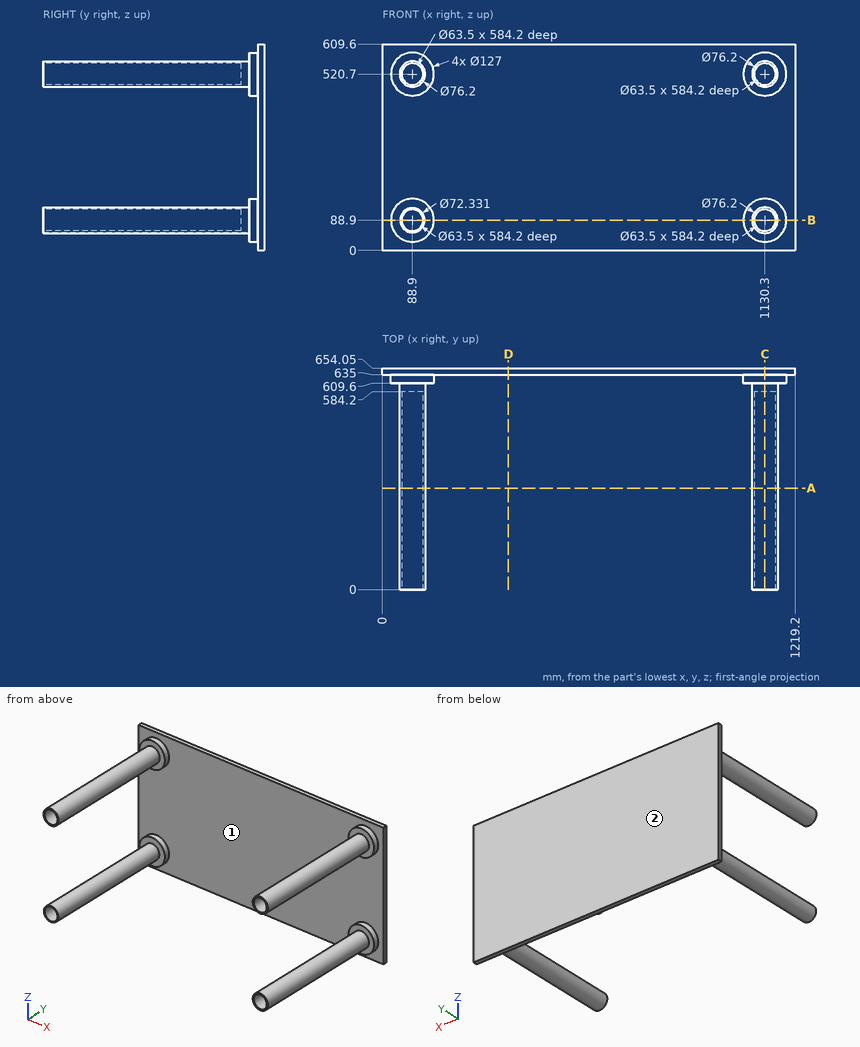
The figure shows three views and two pictorial views of one solid part (mm, origin at its lowest corner). Answer the questions. Coordinates: 2 decimals unless noted, no trailing zeros. Write each loop counter-clockwise with the first axis right and the second up, starting at its lowest first coordinate (ties: lowest second). Pieces come first, ordered by that corner, then holes. Notation, with made-up numbers: (74.5, 47) -> (82.5, 47) arc R14 cw to (82.5, 54) -> close; hole circle Ø10 at (52.25, 24). An arc over 180 degrees is marked (long way). Return JSON: item names as keys, results as strings.
(1) Consider line 1 along X through (y, z) = (209, 520); line 2 along Z through (x, y) = (88, 160); line 3 along Z through (x, y) = (1130.3, 406). Determine where each line is inside the solid, lowest interval first. Write a range as from..to.
Answers below:
{"line 1": "50.81..57.16, 120.64..126.99, 1092.21..1098.56, 1162.04..1168.39", "line 2": "52.75..57.16, 120.64..125.05, 482.61..488.96, 552.44..558.79", "line 3": "50.8..57.15, 120.65..127, 482.6..488.95, 552.45..558.8"}
(2) For a pull along X with two mould halves and no side action, classify the marked faces 1 and 2 as pulls with the +X half, pulls with the -X half, needs draft (parallel to the pull), parting line crosses it, or undercut.
Answers below:
{"face 1": "undercut", "face 2": "needs draft"}
(3) The part is cut by section C-C on x = 1130.3. Give the vertices of the cut face in (y, z), then the cut area to 3 significant figures.
Answers below:
{"outline": "(0, 50.8) -> (609.6, 50.8) -> (609.6, 25.4) -> (635, 25.4) -> (635, 0) -> (654.05, 0) -> (654.05, 609.6) -> (635, 609.6) -> (635, 584.2) -> (609.6, 584.2) -> (609.6, 558.8) -> (0, 558.8) -> (0, 552.45) -> (584.2, 552.45) -> (584.2, 488.95) -> (0, 488.95) -> (0, 482.6) -> (609.6, 482.6) -> (609.6, 457.2) -> (635, 457.2) -> (635, 152.4) -> (609.6, 152.4) -> (609.6, 127) -> (0, 127) -> (0, 120.65) -> (584.2, 120.65) -> (584.2, 57.15) -> (0, 57.15) -> close", "area": "36,800 mm^2"}
(4) The part is cut by section A-A on y = 300. Give the vertices of the cut face in (x, z), then the cut area to 3 significant figures.
Answers below:
{"outline": "circle Ø76.2 at (88.9, 520.7); circle Ø72.33 at (88.9, 88.9); circle Ø76.2 at (1130.3, 88.9); circle Ø76.2 at (1130.3, 520.7); hole circle Ø63.5 at (88.9, 88.9); hole circle Ø63.5 at (88.9, 520.7); hole circle Ø63.5 at (1130.3, 88.9); hole circle Ø63.5 at (1130.3, 520.7)", "area": "5,120 mm^2"}
(5) The part is cut by section D-D on x = 372. Give the vertices of the cut face in (y, z), then the cut area to 3 significant figures.
Answers below:
{"outline": "(635, 0) -> (654.05, 0) -> (654.05, 609.6) -> (635, 609.6) -> close", "area": "11,600 mm^2"}
(6) Each of these flat-tipped pins is pushed along its axis until it touches: P1, Ø19, axis at x = 103, z = 524.5, coming from the -Y side; P2, Ø6, axis at y = 190, z = 524.5, coming from the +X side; P3, Ø2, axis at x = 949.5, z = 217, coming from the -Y side. Where does it stop, or does it pass through?
Answers below:
{"P1": "y = 584.2", "P2": "x = 1168.39", "P3": "y = 635"}
(7) The part is cut by section B-B on z = 88.9. Give the vertices of the cut face in (x, y).
Answers below:
{"outline": "(0, 635) -> (25.4, 635) -> (25.4, 609.6) -> (52.73, 609.6) -> (52.73, 0) -> (57.15, 0) -> (57.15, 584.2) -> (120.65, 584.2) -> (120.65, 0) -> (125.07, 0) -> (125.07, 609.6) -> (152.4, 609.6) -> (152.4, 635) -> (1066.8, 635) -> (1066.8, 609.6) -> (1092.2, 609.6) -> (1092.2, 0) -> (1098.55, 0) -> (1098.55, 584.2) -> (1162.05, 584.2) -> (1162.05, 0) -> (1168.4, 0) -> (1168.4, 609.6) -> (1193.8, 609.6) -> (1193.8, 635) -> (1219.2, 635) -> (1219.2, 654.05) -> (0, 654.05) -> close"}
